CAD build for the part. Positions are in the model's coordinates, mm. Give positions to 0.01 mm unless a question says otherwise; leave off trailing zeros. Write each loop counter-clockwise with the first axis right and the second up, starting at its lowest first coordinate (ties: lowest second). Pieces come first, ordered by that corner, then holes. Notation, with made-up numbers: M -14,12.25 L -6,12.25 A14 ccw -6,23.25 Z; hole C 72.25,85 d10. An arc over 180 degrees is marked long. One line per question, with ' | ' between items. Start each with the question number.
1. Cut at A-A, the plane y = 85. Write the cut outline in (x, z).
2. Cut at C-C, the plane z = -0.65. Count the separate pieces of the cut face and the enclosed holes in it, then the cut area to 3 significant figures.
3. Cut at D-D, the plane y = -82.5. Write the cut outline in (x, z), then the cut area to 3 significant figures.
4. Cut at B-B, the plane x = -59. Write the cut outline in (y, z), then the cut area to 3 significant figures.
5. Wall check: L1, parallel to X at y = 7, z = 0.85; L2, parallel to Y at x = 32, z = 0.25; L3, parallel to Y at x = -69, z = 0.1. Give the ranges that are in metal, low to high.
6. Flat gauge pins, fed straight in: pin 1 (1.5 mm diameter, centred on x = 5.5, z = -1, fed in from +Y); pin 2 (0.9 mm diameter, centred on x = 0, z = 0, fed in from -Y). Where does each tip first touch, or does it go through?
```python
from build123d import *

# Parameters (mm, degrees)
MODEL_R             = 1.6
MODEL_R_2           = 15
MODEL_R_3           = 11
MODEL_R_4           = 7.5
BOSS_EXTRUDE1_DEPTH = 1.5


with BuildPart() as part:
    # Model → Boss-Extrude1 (new, symmetric)
    with BuildSketch(Plane.XY):
        with BuildLine():
            Line((-87, -128), (-54, -128))
            ThreePointArc((-54, -128), (-51.171572875, -126.828427125), (-50, -124))
            Line((-50, -124), (-50, -115.5))
            ThreePointArc((-50, -115.5), (-48.828427125, -112.671572875), (-46, -111.5))
            Line((-46, -111.5), (46, -111.5))
            ThreePointArc((46, -111.5), (48.828427125, -112.671572875), (50, -115.5))
            Line((50, -115.5), (50, -124))
            ThreePointArc((50, -124), (51.171572875, -126.828427125), (54, -128))
            Line((54, -128), (87, -128))
            ThreePointArc((87, -128), (90.535533906, -126.535533906), (92, -123))
            Line((92, -123), (92, 123))
            ThreePointArc((92, 123), (90.535533906, 126.535533906), (87, 128))
            Line((87, 128), (54, 128))
            ThreePointArc((54, 128), (51.171572875, 126.828427125), (50, 124))
            Line((50, 124), (50, 115.5))
            ThreePointArc((50, 115.5), (48.828427125, 112.671572875), (46, 111.5))
            Line((46, 111.5), (-46, 111.5))
            ThreePointArc((-46, 111.5), (-48.828427125, 112.671572875), (-50, 115.5))
            Line((-50, 115.5), (-50, 124))
            ThreePointArc((-50, 124), (-51.171572875, 126.828427125), (-54, 128))
            Line((-54, 128), (-87, 128))
            ThreePointArc((-87, 128), (-90.535533906, 126.535533906), (-92, 123))
            Line((-92, 123), (-92, -123))
            ThreePointArc((-92, -123), (-90.535533906, -126.535533906), (-87, -128))
        make_face()
        with Locations((-75, 115)):
            Circle(MODEL_R, mode=Mode.SUBTRACT)
        with Locations((75, 115)):
            Circle(MODEL_R, mode=Mode.SUBTRACT)
        with Locations((-75, -115)):
            Circle(MODEL_R, mode=Mode.SUBTRACT)
        with Locations((75, -115)):
            Circle(MODEL_R, mode=Mode.SUBTRACT)
        with Locations((-69, 88.5)):
            Circle(MODEL_R_2, mode=Mode.SUBTRACT)
        with Locations((69, 88.5)):
            Circle(MODEL_R_2, mode=Mode.SUBTRACT)
        with Locations((-69, -88.5)):
            Circle(MODEL_R_2, mode=Mode.SUBTRACT)
        with Locations((69, -88.5)):
            Circle(MODEL_R_2, mode=Mode.SUBTRACT)
        with Locations((-24.5, 44.5)):
            Circle(MODEL_R, mode=Mode.SUBTRACT)
        with Locations((24.5, 44.5)):
            Circle(MODEL_R, mode=Mode.SUBTRACT)
        with Locations((-24.5, 102.5)):
            Circle(MODEL_R, mode=Mode.SUBTRACT)
        with Locations((24.5, 102.5)):
            Circle(MODEL_R, mode=Mode.SUBTRACT)
        with Locations((0, -88.5)):
            Circle(MODEL_R_3, mode=Mode.SUBTRACT)
        with Locations((-76.5, -57)):
            Circle(MODEL_R, mode=Mode.SUBTRACT)
        with Locations((-76.5, 57)):
            Circle(MODEL_R, mode=Mode.SUBTRACT)
        with Locations((76.5, -57)):
            Circle(MODEL_R, mode=Mode.SUBTRACT)
        with Locations((76.5, 57)):
            Circle(MODEL_R, mode=Mode.SUBTRACT)
        with Locations((-32.5, -88.5)):
            Circle(MODEL_R_3, mode=Mode.SUBTRACT)
        with Locations((32.5, -88.5)):
            Circle(MODEL_R_3, mode=Mode.SUBTRACT)
        with Locations((-42, 81)):
            Circle(MODEL_R_4, mode=Mode.SUBTRACT)
        with Locations((42, 81)):
            Circle(MODEL_R_4, mode=Mode.SUBTRACT)
        with BuildLine():
            Line((-24.5, 40.5), (-13.6, 40.5))
            ThreePointArc((-13.6, 40.5), (-12.46862915, 40.03137085), (-12, 38.9))
            Line((-12, 38.9), (-12, -59.4))
            ThreePointArc((-12, -59.4), (-12.46862915, -60.53137085), (-13.6, -61))
            Line((-13.6, -61), (-68.5, -61))
            ThreePointArc((-68.5, -61), (-71.328427125, -59.828427125), (-72.5, -57))
            ThreePointArc((-72.5, -57), (-73.671572875, -54.171572875), (-76.5, -53))
            ThreePointArc((-76.5, -53), (-79.328427125, -51.828427125), (-80.5, -49))
            Line((-80.5, -49), (-80.5, 49))
            ThreePointArc((-80.5, 49), (-79.328427125, 51.828427125), (-76.5, 53))
            ThreePointArc((-76.5, 53), (-73.671572875, 54.171572875), (-72.5, 57))
            ThreePointArc((-72.5, 57), (-71.328427125, 59.828427125), (-68.5, 61))
            Line((-68.5, 61), (-32.5, 61))
            ThreePointArc((-32.5, 61), (-29.671572875, 59.828427125), (-28.5, 57))
            Line((-28.5, 57), (-28.5, 44.5))
            ThreePointArc((-28.5, 44.5), (-27.328427125, 41.671572875), (-24.5, 40.5))
        make_face(mode=Mode.SUBTRACT)
        with BuildLine():
            Line((28.5, 44.5), (28.5, 57))
            ThreePointArc((28.5, 57), (29.671572875, 59.828427125), (32.5, 61))
            Line((32.5, 61), (68.5, 61))
            ThreePointArc((68.5, 61), (71.328427125, 59.828427125), (72.5, 57))
            ThreePointArc((72.5, 57), (73.671572875, 54.171572875), (76.5, 53))
            ThreePointArc((76.5, 53), (79.328427125, 51.828427125), (80.5, 49))
            Line((80.5, 49), (80.5, -49))
            ThreePointArc((80.5, -49), (79.328427125, -51.828427125), (76.5, -53))
            ThreePointArc((76.5, -53), (73.671572875, -54.171572875), (72.5, -57))
            ThreePointArc((72.5, -57), (71.328427125, -59.828427125), (68.5, -61))
            Line((68.5, -61), (13.6, -61))
            ThreePointArc((13.6, -61), (12.46862915, -60.53137085), (12, -59.4))
            Line((12, -59.4), (12, 38.9))
            ThreePointArc((12, 38.9), (12.46862915, 40.03137085), (13.6, 40.5))
            Line((13.6, 40.5), (24.5, 40.5))
            ThreePointArc((24.5, 40.5), (27.328427125, 41.671572875), (28.5, 44.5))
        make_face(mode=Mode.SUBTRACT)
        with BuildLine():
            Line((-16.5, 48.5), (16.5, 48.5))
            ThreePointArc((16.5, 48.5), (19.328427125, 49.671572875), (20.5, 52.5))
            Line((20.5, 52.5), (20.5, 94.5))
            ThreePointArc((20.5, 94.5), (19.328427125, 97.328427125), (16.5, 98.5))
            Line((16.5, 98.5), (-16.5, 98.5))
            ThreePointArc((-16.5, 98.5), (-19.328427125, 97.328427125), (-20.5, 94.5))
            Line((-20.5, 94.5), (-20.5, 52.5))
            ThreePointArc((-20.5, 52.5), (-19.328427125, 49.671572875), (-16.5, 48.5))
        make_face(mode=Mode.SUBTRACT)
        with BuildLine():
            Line((-6, 23.1), (6, 23.1))
            ThreePointArc((6, 23.1), (7.6, 21.5), (6, 19.9))
            Line((6, 19.9), (-6, 19.9))
            ThreePointArc((-6, 19.9), (-7.6, 21.5), (-6, 23.1))
        make_face(mode=Mode.SUBTRACT)
        with BuildLine():
            Line((-6, -19.9), (6, -19.9))
            ThreePointArc((6, -19.9), (7.6, -21.5), (6, -23.1))
            Line((6, -23.1), (-6, -23.1))
            ThreePointArc((-6, -23.1), (-7.6, -21.5), (-6, -19.9))
        make_face(mode=Mode.SUBTRACT)
        with BuildLine():
            Line((-6, 17.5), (6, 17.5))
            ThreePointArc((6, 17.5), (7.13137085, 17.03137085), (7.6, 15.9))
            Line((7.6, 15.9), (7.6, -15.9))
            ThreePointArc((7.6, -15.9), (7.13137085, -17.03137085), (6, -17.5))
            Line((6, -17.5), (-6, -17.5))
            ThreePointArc((-6, -17.5), (-7.13137085, -17.03137085), (-7.6, -15.9))
            Line((-7.6, -15.9), (-7.6, 15.9))
            ThreePointArc((-7.6, 15.9), (-7.13137085, 17.03137085), (-6, 17.5))
        make_face(mode=Mode.SUBTRACT)
        with BuildLine():
            Line((-6, 25.5), (6, 25.5))
            ThreePointArc((6, 25.5), (7.13137085, 25.96862915), (7.6, 27.1))
            Line((7.6, 27.1), (7.6, 38.9))
            ThreePointArc((7.6, 38.9), (7.13137085, 40.03137085), (6, 40.5))
            Line((6, 40.5), (-6, 40.5))
            ThreePointArc((-6, 40.5), (-7.13137085, 40.03137085), (-7.6, 38.9))
            Line((-7.6, 38.9), (-7.6, 27.1))
            ThreePointArc((-7.6, 27.1), (-7.13137085, 25.96862915), (-6, 25.5))
        make_face(mode=Mode.SUBTRACT)
        with BuildLine():
            Line((-6, -25.5), (6, -25.5))
            ThreePointArc((6, -25.5), (7.13137085, -25.96862915), (7.6, -27.1))
            Line((7.6, -27.1), (7.6, -59.4))
            ThreePointArc((7.6, -59.4), (7.13137085, -60.53137085), (6, -61))
            Line((6, -61), (-6, -61))
            ThreePointArc((-6, -61), (-7.13137085, -60.53137085), (-7.6, -59.4))
            Line((-7.6, -59.4), (-7.6, -27.1))
            ThreePointArc((-7.6, -27.1), (-7.13137085, -25.96862915), (-6, -25.5))
        make_face(mode=Mode.SUBTRACT)
    extrude(amount=BOSS_EXTRUDE1_DEPTH, both=True)


solid = part.part
```
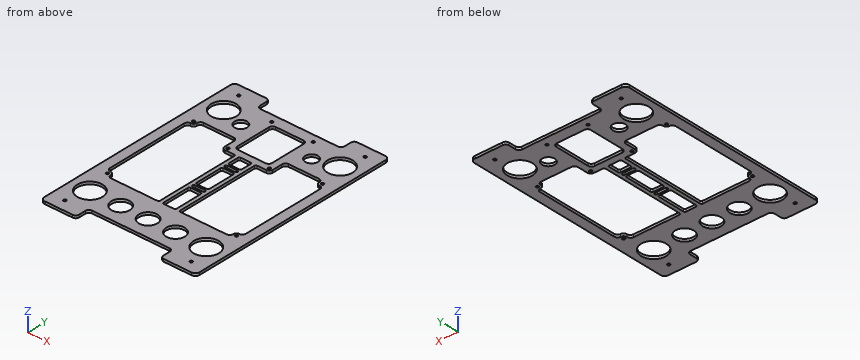
Here are the results:
1) outline: M -92,-1.5 L -83.59,-1.5 L -83.59,1.5 L -92,1.5 Z; M -54.41,-1.5 L -48.34,-1.5 L -48.34,1.5 L -54.41,1.5 Z; M -35.66,-1.5 L -20.5,-1.5 L -20.5,1.5 L -35.66,1.5 Z; M 20.5,-1.5 L 35.66,-1.5 L 35.66,1.5 L 20.5,1.5 Z; M 48.34,-1.5 L 54.41,-1.5 L 54.41,1.5 L 48.34,1.5 Z; M 83.59,-1.5 L 92,-1.5 L 92,1.5 L 83.59,1.5 Z
2) separate pieces: 1 | enclosed holes: 29 | area: 20,200 mm^2
3) outline: M -92,-1.5 L -82.75,-1.5 L -82.75,1.5 L -92,1.5 Z; M -55.25,-1.5 L -41.72,-1.5 L -41.72,1.5 L -55.25,1.5 Z; M -23.28,-1.5 L -9.22,-1.5 L -9.22,1.5 L -23.28,1.5 Z; M 9.22,-1.5 L 23.28,-1.5 L 23.28,1.5 L 9.22,1.5 Z; M 41.72,-1.5 L 55.25,-1.5 L 55.25,1.5 L 41.72,1.5 Z; M 82.75,-1.5 L 92,-1.5 L 92,1.5 L 82.75,1.5 Z | area: 221 mm^2
4) outline: M -128,-1.5 L -99.68,-1.5 L -99.68,1.5 L -128,1.5 Z; M -77.32,-1.5 L -61,-1.5 L -61,1.5 L -77.32,1.5 Z; M 61,-1.5 L 77.32,-1.5 L 77.32,1.5 L 61,1.5 Z; M 99.68,-1.5 L 128,-1.5 L 128,1.5 L 99.68,1.5 Z | area: 268 mm^2
5) L1: -92 to -80.5, -12 to -7.6, 7.6 to 12, 80.5 to 92 | L2: -111.5 to -99.49, -77.51 to -61, 60.97 to 111.5 | L3: -128 to -103.5, -73.5 to -60.97, 60.97 to 73.5, 103.5 to 128
6) pin 1: y = 111.5 | pin 2: y = -111.5
